Read the model definition and answer for the solid it produces. Units are mm, in the model's axes. Face numbers are marked on the shaded views. A direction names the side the tool comes from. Coordinates: 2 decimals unless noted, no trailing zeros. Write each loop counter-clockwise with the first axis right and the second up, starting at its lowest first coordinate (ties: lowest second). Pieces come first, ordered by that corner, then holes. Notation, with made-up numbers: (65.25, -33) -> (73.25, -33) arc R15 ccw to (73.25, -11) -> close; hole circle Ø9 at (25, 63). An arc over 180 degrees is marked (long way). One line per item, written item: value. Start each with the question number.
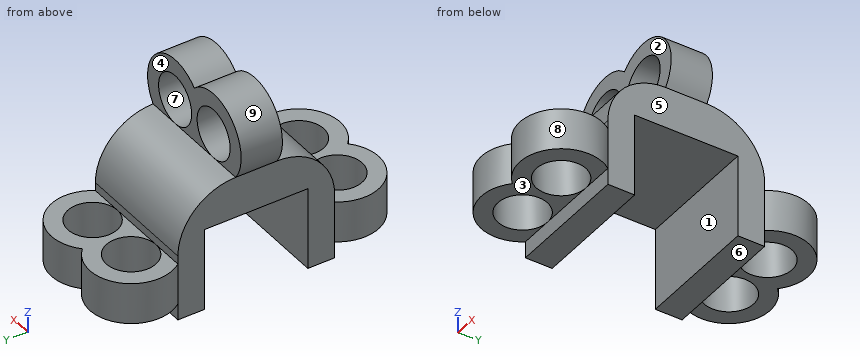
Autodesk Fusion 360 part; units mm, degrees
sketch "Sketch1" plane through (0, 0, 0) normal (0, 0, 1) x (1, 0, 0)
  line L0 (7.5, -9.5) -> (-7.5, -9.5)
  line L1 (-7.5, -9.5) -> (-7.5, 9.5)
  line L2 (-7.5, 9.5) -> (7.5, 9.5)
  line L3 (7.5, 9.5) -> (7.5, -9.5)
  line L4 (7.5, -9.5) -> (-7.5, 9.5) construction
  line L5 (-7.5, -9.5) -> (7.5, 9.5) construction
  dimension "d1" = 15
  dimension "d2" = 19
extrude "Extrude1" add sketch "Sketch1" against normal blind 15
sketch "Sketch2" plane through (0, 0, -15) normal (0, 0, -1) x (1, 0, 0)
  line L0 (-7.5, -9.5) -> (7.5, -9.5)
  line L1 (7.5, -9.5) -> (7.5, 9.5)
  line L2 (7.5, 9.5) -> (-7.5, 9.5)
  line L3 (-7.5, 9.5) -> (-7.5, -9.5)
  line L4 (7.5, 6.25) -> (-7.5, 6.25)
  line L5 (-7.5, 6.25) -> (-7.5, -6.25)
  line L6 (-7.5, -6.25) -> (7.5, -6.25)
  line L7 (7.5, -6.25) -> (7.5, 6.25)
  line L8 (7.5, 6.25) -> (-7.5, -6.25) construction
  line L9 (-7.5, 6.25) -> (7.5, -6.25) construction
  dimension "d5" = 15
  dimension "d6" = 12.5
extrude "Extrude2" cut sketch "Sketch2" against normal blind 10 contours L1 L3 L4 L5 L6 L7
fillet "Fillet1" radius 7 2 edges at (0, 9.5, 0) (0, -9.5, 0)
ref_plane "WorkPlane1" through (0, 0, 0) normal (0, 1, 0) x (0, 0, 1)
sketch "Sketch4" plane through (0, 0, 0) normal (0, 1, 0) x (1, 0, 0)
  line L0 (-7.5, 0) -> (-7.5, 7)
  line L1 (7.5, 7) -> (7.5, 0)
  line L2 (7.5, 0) -> (-7.5, 0)
  line L3 (-7.5, 7) -> (-7.5, 15)
  line L4 (7.5, 15) -> (-7.5, 15)
  line L5 (7.5, 7) -> (7.5, 15)
  line L6 (0, 0) -> (-3.5, 0) construction
  line L7 (0, 0) -> (3.5, 0) construction
  line L8 (-3.5, 0) -> (-3.5, -3) construction
  line L9 (3.5, 0) -> (3.5, -3) construction
  circle A0 centre (3.5, -3) radius 3
  circle A1 centre (-3.5, -3) radius 3
  circle A2 centre (-3.5, -3) radius 5
  circle A3 centre (3.5, -3) radius 5
  dimension "d20" = 3.5
  dimension "d21" = 3.5
  dimension "d22" = 3
  dimension "d23" = 3
  dimension "d24" = 6
  dimension "d25" = 6
  dimension "d26" = 10
  dimension "d27" = 10
extrude "Extrude3" add sketch "Sketch4" along normal mid plane 5 contours L2 A2 A3 | L2 A1 A2 A3 | L2 A1 A3 | L2 A2 A3 | L2 A0 A1 A2 A3 | L2 A0 A2 A3 | L2 A0 A2 picked at (-1.7132, 0.4693) picked at (1.7132, 0.4693)
ref_plane "WorkPlane2" through (0, 0, -8) normal (0, 0, 1) x (1, 0, 0)
sketch "Sketch5" plane through (0, 0, -8) normal (0, 0, 1) x (1, 0, 0)
  line L0 (-7.5, 6.25) -> (-7.5, 9.5)
  line L1 (-7.5, -9.5) -> (-7.5, -6.25)
  line L2 (-7.5, 9.5) -> (7.5, 9.5)
  line L3 (7.5, 9.5) -> (7.5, 6.25)
  line L4 (7.5, -6.25) -> (7.5, -9.5)
  line L5 (7.5, -9.5) -> (-7.5, -9.5)
  line L6 (0, 9.5) -> (-3.5, 9.5) construction
  line L7 (0, 9.5) -> (3.5, 9.5) construction
  line L8 (-3.5, 9.5) -> (-3.5, 12.5) construction
  line L9 (3.5, 9.5) -> (3.5, 12.5) construction
  line L10 (10.0516, 0) -> (-10.1091, 0) construction
  circle A0 centre (3.5, 12.5) radius 3
  circle A1 centre (-3.5, 12.5) radius 3
  circle A2 centre (-3.5, 12.5) radius 5
  circle A3 centre (3.5, 12.5) radius 5
  circle A4 centre (3.5, -12.5) radius 5
  circle A5 centre (3.5, -12.5) radius 3
  circle A6 centre (-3.5, -12.5) radius 5
  circle A7 centre (-3.5, -12.5) radius 3
  line L11 (8.5, 2.5) -> (7.5, 2.5)
  line L12 (7.5, -2.5) -> (8.5, -2.5)
  line L13 (7.5, -6.25) -> (7.5, -2.5)
  line L14 (7.5, 2.5) -> (7.5, 6.25)
  line L15 (8.5, 2.5) -> (8.5, -2.5)
  line L16 (-7.5, 2.5) -> (-8.5, 2.5)
  line L17 (-8.5, -2.5) -> (-7.5, -2.5)
  line L18 (-7.5, 6.25) -> (-7.5, 2.5)
  line L19 (-7.5, -2.5) -> (-7.5, -6.25)
  line L20 (-8.5, 2.5) -> (-8.5, -2.5)
  dimension "d31" = 3.5
  dimension "d32" = 3.5
  dimension "d33" = 3
  dimension "d34" = 3
  dimension "d35" = 6
  dimension "d36" = 6
  dimension "d37" = 10
  dimension "d38" = 10
extrude "Extrude4" add sketch "Sketch5" against normal blind 5 contours L2 A1 A2 A3 | L2 A1 A3 | L2 A0 A2 A3 | L2 A0 A1 A2 A3 | L2 A0 A2 | L5 A4 A6 A7 | L5 A4 A7 | L5 A4 A5 A6 | L5 A4 A5 A6 A7 | L5 A5 A6
equation "d2 = 13 mm + 3 mm + 3 mm"
1. A cutting plane is placed at B-B on y = 12.5. Give the vertices of the cut face in (x, z), then the cut area to 3 significant figures.
2. A cutting plane is placed at D-D on z = -9. Give the vertices of the cut face in (x, y), then the cut area to 3 significant figures.
3. Given pin 1 (0.6 mm diameter, centred on x = 1.5, z = -14, fed in from +Y); pin 2 (5 mm diameter, centred on x = 6.5, z = -0.5, fed in from +Y); pin 3 (2.5 mm diameter, centred on x = -1.5, z = 5.5, fed in from +Y), each flat-ended and moving along its own axis, determine where each tip first touches the part or whether it passes through.
4. For a pull along Z with two mould halves and no side action, classify the marked faces 6, 7, 8 and 9 as +Z half, -Z half, draft (parallel to the pull), parting line (faces both ways), or undercut.
5. Find the intervals of material crossed by probe 1 along X at (y, z) = (-12.5, -11.5); probe 2 along Y at (x, z) = (-3.5, -11); probe 3 along Y at (x, z) = (1.75, -12), in increasing order. Write a range as from..to.
6. A tool of negligible diameter and unlimited length cuts with its end or side. For the marked faces 1, 2, 3, 4 and 5, from which of +Z, -Z, +X, -X, +Y, -Y can it reach the whole face along a straight path? Write none if from no direction.
7. A cutting plane is placed at C-C on x = -3. Count the separate pieces of the cut face and the enclosed holes in it, then the cut area to 3 significant figures.
8. A cutting plane is placed at A-A on z = 3. Give the vertices of the cut face in (x, y).
Derived:
1. outline: (-8.5, -13) -> (-6.5, -13) -> (-6.5, -8) -> (-8.5, -8) -> close; (-0.5, -13) -> (0.5, -13) -> (0.5, -8) -> (-0.5, -8) -> close; (6.5, -13) -> (8.5, -13) -> (8.5, -8) -> (6.5, -8) -> close
1. area: 25.0 mm2
2. outline: (-7.5, -9.5) arc R5 ccw to (0, -16.07) arc R5 ccw to (7.5, -9.5) -> (7.5, -6.25) -> (-7.5, -6.25) -> close; (-7.5, 6.25) -> (7.5, 6.25) -> (7.5, 9.5) arc R5 ccw to (0, 16.07) arc R5 ccw to (-7.5, 9.5) -> close; hole circle Ø6 at (-3.5, -12.5); hole circle Ø6 at (-3.5, 12.5); hole circle Ø6 at (3.5, -12.5); hole circle Ø6 at (3.5, 12.5)
2. area: 225 mm2
3. pin 1: stops at y = 9.5
3. pin 2: stops at y = 8.24
3. pin 3: stops at y = 2.5
4. face 6: -Z half
4. face 7: undercut
4. face 8: draft
4. face 9: parting line
5. probe 1: x = -8.5..-6.5, -0.5..0.5, 6.5..8.5
5. probe 2: y = -17.5..-15.5, -9.5..-6.25, 6.25..9.5, 15.5..17.5
5. probe 3: y = -17.18..-14.94, -10.06..-6.25, 6.25..10.06, 14.94..17.18
6. face 1: -Z, +X, -X
6. face 2: +Z, +X, -X, -Y
6. face 3: -Z, +X, -X, -Y
6. face 4: +Z, +X, -X, +Y
6. face 5: -Z, +X
7. separate pieces: 4
7. enclosed holes: 0
7. area: 170 mm2
8. outline: (-8.5, -2.5) -> (-6.5, -2.5) -> (-6.5, 2.5) -> (-8.5, 2.5) -> close; (-0.5, -2.5) -> (0.5, -2.5) -> (0.5, 2.5) -> (-0.5, 2.5) -> close; (6.5, -2.5) -> (8.5, -2.5) -> (8.5, 2.5) -> (6.5, 2.5) -> close
